The listing builds one solid part. Answer for the finished solid, in the listing's coordinates (mm). Face numbers are marked on the shaded views. Give positions to 0.01 mm unless a question says otherwise; leave off trailing zeros. Order: outer loops, then holes, each group sorted by start corner. A loop starts at its lowest first (then second) coordinate and runs counter-clockwise, first axis right, second up. Notation, with made-up numbers: (-30, -35) - (-4, -35) arc R32 cw to (-4, -9) - close; hole circle Ø7 at (-16, 25.25). An arc over 180 degrees is marked (long way). Use a Markdown table: item, result. Add a question column.
1) Flat-ended cylindrical pins translate along their axes: pin 1 (1 mm diameter, centred on x = -151.5, z = 27.5, fed in from -Y); pin 2 (3 mm diameter, centred on y = -84, z = 33, fed in from -X) (3 decimals); pin 3 (8.5 mm diameter, centred on x = -97, z = 19.5, fed in from +Y). Find the tip coordinate at first contact, or state that the pin passes through.
2) The mould has two halves that part along Z. Classify the marked faces 1, 2, 3 and 4: released by +Z, released by -Z, zero draft, split by the parting line, or undercut.
3) Find section C-C, the plane z = 17.5. Determine the outline of the cut face in (x, y).
4) Straight lines are drawn through the part: line 1 (Z direction, x = -180, y = -127.5); line 2 (X direction, y = -8, z = 21); line 3 (Y direction, x = -38.5, z = 20). For each, find the intervals that lie inside material, in ascending order.
5) Find section D-D, the plane z = 30.5. Determine the outline of the cut face in (x, y).
6) Find section A-A, the plane y = -22. Determine the outline of the cut face in (x, z).
7) Find section B-B, the plane x = -90.5. Determine the outline of the cut face in (y, z).
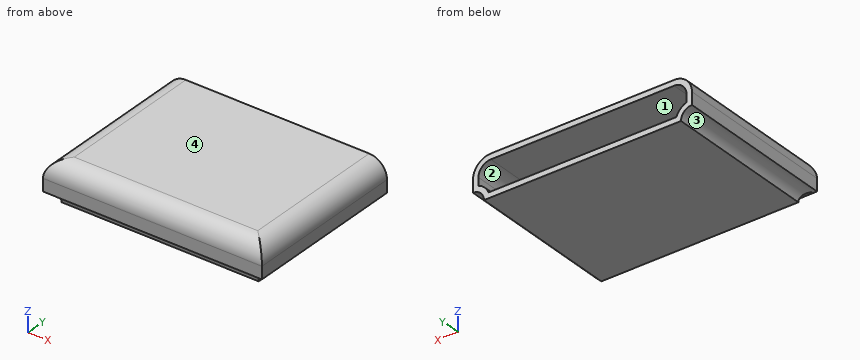
from build123d import *

# Parameters (mm, degrees)
F5_DEPTH = 152.4
F1_R     = 10.16
F2_DEPTH = 254
F3_R     = 16.51
F6_T     = -5.08


with BuildPart() as f5:
    # F0 (on Front) → F5 (new body)
    with BuildSketch(Plane.XZ):
        with BuildLine():
            Line((-193.04, 0), (-10.16, 0))
            ThreePointArc((-10.16, 0), (-7.184205, 7.184205), (0, 10.16))
            Line((0, 10.16), (0, 38.1))
            Line((0, 38.1), (-203.2, 38.1))
            Line((-203.2, 38.1), (-203.2, 10.16))
            ThreePointArc((-203.2, 10.16), (-196.015795, 7.184205), (-193.04, 0))
        make_face()
    extrude(amount=F5_DEPTH)

    # F1 (on face) → F2 (cut)
    with BuildSketch(Plane.YZ):
        with Locations((-153.180798, 0)):
            Circle(F1_R)
    extrude(amount=-F2_DEPTH, mode=Mode.SUBTRACT)

    # F3
    f3_edges = [f5.edges().sort_by_distance(p)[0] for p in [
        (-101.6, -152.4, 38.1),
        (-203.2, -76.2, 38.1),
        (0, -76.2, 38.1),
    ]]
    fillet(f3_edges, radius=F3_R)

    # F6
    f6_openings = [f5.faces().sort_by_distance(p)[0] for p in [
        (-101.6, 0, 19.129387),
    ]]
    offset(amount=F6_T, openings=f6_openings)


solid = f5.part
The answers:
| question | item | result |
|---|---|---|
| 1 | pin 1 | y = -151.49 |
| 1 | pin 2 | x = -199.895 |
| 1 | pin 3 | y = -147.11 |
| 2 | face 1 | undercut |
| 2 | face 2 | undercut |
| 2 | face 3 | released by -Z |
| 2 | face 4 | released by +Z |
| 3 | outline | (-203.2, -152.4) - (0, -152.4) - (0, 0) - (-5.08, 0) - (-5.08, -147.32) - (-198.12, -147.32) - (-198.12, 0) - (-203.2, 0) - close |
| 4 | line 1 | 0 to 5.08, 33.02 to 38.1 |
| 4 | line 2 | -203.2 to -198.12, -5.08 to 0 |
| 4 | line 3 | -152.4 to -147.32 |
| 5 | outline | (-200.59, -149.79) - (-2.61, -149.79) - (-2.61, 0) - (-9.35, 0) - (-9.35, -143.05) - (-193.85, -143.05) - (-193.85, 0) - (-200.59, 0) - close |
| 6 | outline | (-203.2, 10.16) arc R10.16 cw to (-193.04, 0) - (-10.16, 0) arc R10.16 cw to (0, 10.16) - (0, 21.59) arc R16.51 ccw to (-16.51, 38.1) - (-186.69, 38.1) arc R16.51 ccw to (-203.2, 21.59) - close; hole (-198.12, 14.37) arc R15.24 cw to (-188.83, 5.08) - (-14.37, 5.08) arc R15.24 cw to (-5.08, 14.37) - (-5.08, 21.59) arc R11.43 ccw to (-16.51, 33.02) - (-186.69, 33.02) arc R11.43 ccw to (-198.12, 21.59) - close |
| 7 | outline | (-152.4, 10.13) arc R10.16 cw to (-143.02, 0) - (0, 0) - (0, 5.08) - (-138.81, 5.08) arc R15.24 ccw to (-147.32, 14.07) - (-147.32, 21.59) arc R11.43 cw to (-135.89, 33.02) - (0, 33.02) - (0, 38.1) - (-135.89, 38.1) arc R16.51 ccw to (-152.4, 21.59) - close |
